Autodesk Inventor part; units mm, degrees
ref_plane "YZ Plane" through (0, 0, 0) normal (1, 0, 0) x (0, 1, 0)
ref_plane "XZ Plane" through (0, 0, 0) normal (0, 1, 0) x (-1, 0, 0)
ref_plane "XY Plane" through (0, 0, 0) normal (0, 0, 1) x (1, 0, 0)
sketch "Esquisse1" plane through (0, 0, 0) normal (0, 1, 0) x (-1, 0, 0)
  line L0 (-3.1494, 4.7956) -> (0.3506, 4.7956)
  line L1 (0.3506, 4.7956) -> (0.3506, 3.0956)
  line L2 (0.3506, 3.0956) -> (-3.1494, 3.0956)
  line L3 (-3.1494, 3.0956) -> (-3.1494, 4.7956)
  line L4 (-4.0494, 5.6956) -> (1.2506, 5.6956)
  line L5 (1.2506, 5.6956) -> (1.2506, 2.1956)
  line L6 (1.2506, 2.1956) -> (-4.0494, 2.1956)
  line L7 (-4.0494, 2.1956) -> (-4.0494, 5.6956)
  point P0 (0, 0)
  dimension "d0" = 3.5
  dimension "d1" = 1.7
  dimension "d2" = 0.9
  dimension "d3" = 0.9
  dimension "d4" = 0.9
  dimension "d5" = 0.9
extrude "Extrusion1" add sketch "Esquisse1" along normal blind 12
sketch "Esquisse2" plane through (0, 12, 0) normal (0, 1, 0) x (1, 0, 0)
  line L0 (3.1494, -4.7956) -> (-0.3506, -4.7956)
  line L1 (-0.3506, -4.7956) -> (3.1494, -4.7956)
  line L2 (3.1494, -4.7956) -> (3.1494, -3.0956)
  line L3 (3.1494, -3.0956) -> (-0.3506, -3.0956)
  line L4 (-0.3506, -3.0956) -> (-0.3506, -4.7956)
  point P0 (0, 0)
extrude "Extrusion2" add sketch "Esquisse2" against normal blind 2
equation "\"d3\" = d2"
equation "\"d4\" = d2"
equation "\"d5\" = d2"
properties part number "SwitchOnOff"
CAD build for the part. Positions are in the model's coordinates, mm. A direction names the side the tool comes from. Coordinates: 2 decimals unless noted, no trailing zeros. Order: outer loops, then holes, each group sorted by start corner. A loop starts at its lowest first (then second) coordinate and runs counter-clockwise, first axis right, second up. Notation, with made-up numbers: M -20,-23 L -4,-23 A26 ccw -4,11 Z; hole C -39.5,82.5 d1. An arc over 180 degrees is marked long. Write each question's results on one line, items separated by ' | '. Start each with the question number.
Q1. Which spindle directions (+Z, -Z, +X, -X, +Y, -Y) get a long thin tool onto all of the face, cutting with end or side? Do faces 1 (the flat face through (1, 12, 4)), 2 (the flat face through (1, 5, 4.796)). Say none if no direction does.
Q2. Cut at B-B (x = 1.5). List the corners of the cut face in (y, z), then the cut area to 3 significant figures.
Q3. Cut at A-A (y = 4.75). List the corners of the cut face in (x, z).
Q4. Drill centre lines: probe 1 along X at (y, z) = (5.5, 4.3); probe 2 along Z at (x, y) = (2.75, 3); probe 3 along Y at (x, z) = (1.3, 4.05). Where is each one in solid material? Low to high. Write a range as from..to.
Q5. Cut at C-C (z = 3.95). List the corners of the cut face in (x, y), then the cut area to 3 significant figures.
Q6. Pull direction Z, two halves, no side cores. Call faces 3 (the flat face through (3.149, 5, 4)), 4 (the flat face through (1, 6, 5.696)), 5 (the flat face through (4.049, 6, 4)): +Z half, -Z half, draft (parallel to the pull), parting line (faces both ways), or undercut.
Found:
1) face 1: +Z, -Z, +X, -X, +Y | face 2: -Y
2) outline: M 0,2.2 L 12,2.2 L 12,5.7 L 0,5.7 L 0,4.8 L 10,4.8 L 10,3.1 L 0,3.1 Z | area: 25.0 mm²
3) outline: M -1.25,2.2 L 4.05,2.2 L 4.05,5.7 L -1.25,5.7 Z; hole M -0.35,3.1 L 3.15,3.1 L 3.15,4.8 L -0.35,4.8 Z
4) probe 1: -1.25..-0.35, 3.15..4.05 | probe 2: 2.2..3.1, 4.8..5.7 | probe 3: 10..12
5) outline: M -1.25,0 L -0.35,0 L -0.35,10 L 3.15,10 L 3.15,0 L 4.05,0 L 4.05,12 L -1.25,12 Z | area: 28.6 mm²
6) face 3: undercut | face 4: +Z half | face 5: draft
